```python
from build123d import *

# Parameters (mm, degrees)
F1_DEPTH = 0.6


with BuildPart() as f1:
    # F0 (on Top) → F1 (new body)
    with BuildSketch(Plane.XY):
        with BuildLine():
            Line((3.9, 2), (-3.9, 2))
            ThreePointArc((-3.9, 2), (-5.384924, 1.384924), (-6, -0.1))
            ThreePointArc((-6, -0.1), (-5.384924, -1.584924), (-3.9, -2.2))
            Line((-3.9, -2.2), (3.9, -2.2))
            ThreePointArc((3.9, -2.2), (5.384924, -1.584924), (6, -0.1))
            ThreePointArc((6, -0.1), (5.384924, 1.384924), (3.9, 2))
        make_face()
        with BuildLine():
            ThreePointArc((-5, -0.1), (-4.677817, 0.677817), (-3.9, 1))
            Line((-3.9, 1), (-1.6, 1))
            ThreePointArc((-1.6, 1), (-0.822183, 0.677817), (-0.5, -0.1))
            ThreePointArc((-0.5, -0.1), (-0.822183, -0.877817), (-1.6, -1.2))
            Line((-1.6, -1.2), (-3.9, -1.2))
            ThreePointArc((-3.9, -1.2), (-4.677817, -0.877817), (-5, -0.1))
        make_face(mode=Mode.SUBTRACT)
        with BuildLine():
            ThreePointArc((0.5, -0.1), (0.822183, 0.677817), (1.6, 1))
            Line((1.6, 1), (3.9, 1))
            ThreePointArc((3.9, 1), (4.677817, 0.677817), (5, -0.1))
            ThreePointArc((5, -0.1), (4.677817, -0.877817), (3.9, -1.2))
            Line((3.9, -1.2), (1.6, -1.2))
            ThreePointArc((1.6, -1.2), (0.822183, -0.877817), (0.5, -0.1))
        make_face(mode=Mode.SUBTRACT)
    extrude(amount=F1_DEPTH)


solid = f1.part
```
Model file for the job. Use its own axes, mm. Coordinates: 2 decimals unless noted, no trailing zeros. Order: outer loops, then holes, each group sorted by start corner. A loop starts at its lowest first (then second) coordinate and runs counter-clockwise, first axis right, second up. Notation, with made-up numbers: (-27.5, -32) -> (9.5, -32) arc R26 ccw to (9.5, 7) -> close; hole circle Ø2 at (14.5, 2). An arc over 180 degrees is marked (long way). Return JSON: item names as keys, results as strings.
Item 1: Slice it at D-D (x = 4.75). Write the cut outline in (y, z).
Model answer:
{"outline": "(-2.02, 0) -> (-0.8, 0) -> (-0.8, 0.6) -> (-2.02, 0.6) -> close; (0.6, 0) -> (1.82, 0) -> (1.82, 0.6) -> (0.6, 0.6) -> close"}
Item 2: Wall check: line 1 along Y through (x, z) = (-3.5, 0.2); line 2 along X through (y, z) = (0.3, 0.55); line 3 along X through (y, z) = (-0.6, 0.3). Give the ranges that are in metal, low to high. Write a range as from..to.
Model answer:
{"line 1": "y = -2.2..-1.2, 1..2", "line 2": "x = -5.96..-4.92, -0.58..0.58, 4.92..5.96", "line 3": "x = -5.94..-4.88, -0.62..0.62, 4.88..5.94"}
Item 3: Slice it at C-C (y = 0.7). Write the cut outline in (x, z), then the cut area to 3 significant figures.
Model answer:
{"outline": "(-5.84, 0) -> (-4.65, 0) -> (-4.65, 0.6) -> (-5.84, 0.6) -> close; (-0.85, 0) -> (0.85, 0) -> (0.85, 0.6) -> (-0.85, 0.6) -> close; (4.65, 0) -> (5.84, 0) -> (5.84, 0.6) -> (4.65, 0.6) -> close", "area": "2.44 mm²"}
Item 4: Slice it at B-B (z = 0.3). Write the cut outline in (x, y).
Model answer:
{"outline": "(-6, -0.1) arc R2.1 ccw to (-3.9, -2.2) -> (3.9, -2.2) arc R2.1 ccw to (6, -0.1) arc R2.1 ccw to (3.9, 2) -> (-3.9, 2) arc R2.1 ccw to start; hole (-5, -0.1) arc R1.1 ccw to (-3.9, -1.2) -> (-1.6, -1.2) arc R1.1 ccw to (-0.5, -0.1) arc R1.1 ccw to (-1.6, 1) -> (-3.9, 1) arc R1.1 ccw to start; hole (0.5, -0.1) arc R1.1 ccw to (1.6, -1.2) -> (3.9, -1.2) arc R1.1 ccw to (5, -0.1) arc R1.1 ccw to (3.9, 1) -> (1.6, 1) arc R1.1 ccw to start"}
Item 5: Slice it at A-A (x = -2.25). Write the cut outline in (y, z).
Model answer:
{"outline": "(-2.2, 0) -> (-1.2, 0) -> (-1.2, 0.6) -> (-2.2, 0.6) -> close; (1, 0) -> (2, 0) -> (2, 0.6) -> (1, 0.6) -> close"}
